For this review, take the finished solid that the model builds, in its own axes (mm). A direction names the side the tool comes from. Coordinates: 2 decimals unless noted, no trailing zeros. Write each loop counter-clockwise with the first axis right and the second up, starting at its lowest first coordinate (ties: lowest second). Pieces come first, ordered by that corner, then holes. Notation, with made-up numbers: (-36.5, 29.5) - (-28.5, 29.5) arc R19 ccw to (-28.5, 44.5) - close; hole circle Ø5 at (21, -39.75). An arc over 180 degrees is marked (long way). Use one line per item in the form item = value. Start each with the question number.
1) Tool access review of faces 1 (the flat face through (-1, -44, 8.875)), 2 (the flat face through (35, 35, 0)), 3 (the flat face through (-35, 35, 0)): name each direction out of +Z, -Z, +X, -X, +Y, -Y from which nothing blocks a thin tool from reaching the whole face with its end or side.
2) We need section B-B (y = -17.5). Give the boundary of the cut face in (x, z) (3 decimals).
3) We need section D-D (z = 22.5). Give the boundary of the cut face in (x, y) (3 decimals).
4) We need section A-A (x = 25). Give the boundary of the cut face in (y, z) (3 decimals).
5) We need section C-C (y = 17.5). Give the boundary of the cut face in (x, z) (3 decimals), plus the area to 4 significant figures.
6) For L1, parallel to X at y = 29, z = 0; L2, parallel to X at y = 17.5, z = 7.5 (3 decimals); L3, parallel to Y at x = -12, z = 0 (3 decimals), list the stretches that pass through material, from the lowest coordinate up. Write a range as from..to.
7) Mouldability with a two-part tool opening along X and no side actions: class faces 4 (the flat face through (50, -1, 0)), 5 (the cylindrical face through (-22.422, 28.406, -0.338)), 6 (the cylindrical face through (12.59, 80.78, 0.34)) as pulls with the +X half, pulls with the -X half, needs draft (parallel to the pull), parting line crosses it, or undercut.
8) Insertion check: P1, Ø6, axis at x = -25, y = 17.5, coming from the +Z side; P2, Ø1, axis at x = 10.5, z = 11, coming from the -Y side; P3, Ø4, axis at x = 21, z = -19, coming from the +Y side; P4, Ø9, axis at x = 14.5, y = -46.5, coming from the -Z side (3 decimals). Each pin has a flat end and moves straight along its axis. Give the tip position at first contact, or say it passes through.
```python
from build123d import *

# Parameters (mm, degrees)
SKETCH1_W               = 100
SKETCH1_H               = 70
BOSS_EXTRUDE1_DEPTH     = 25
CUT_EXTRUDE1_DEPTH      = 79.89866919
CUT_EXTRUDE1_DEPTH_BACK = 79.89866919
SKETCH2_R               = 4.875
CUT_EXTRUDE2_DEPTH      = 109.857705285
CUT_EXTRUDE2_DEPTH_BACK = 109.857705285
SKETCH3_R               = 4.875
SKETCH4_R               = 2.6
CUT_EXTRUDE4_DEPTH      = 20
SKETCH5_W               = 100
SKETCH5_H               = 17.75
BOSS_EXTRUDE2_DEPTH     = 20
FILLET1_R               = 2
SKETCH6_W               = 5
SKETCH6_H               = 50
BOSS_EXTRUDE3_DEPTH     = 50
CUT_EXTRUDE5_DEPTH      = 110.960291151
CUT_EXTRUDE5_DEPTH_BACK = 110.960291151
SKETCH7_R               = 2.65
FILLET2_R               = 5
FILLET3_R               = 2


with BuildPart() as part:
    # Sketch1 → Boss-Extrude1 (new, symmetric)
    with BuildSketch(Plane.XY):
        Rectangle(SKETCH1_W, SKETCH1_H)
    extrude(amount=BOSS_EXTRUDE1_DEPTH, both=True)

    # Sketch2 → Cut-Extrude1 (cut, two sides: drawn at the far end of the back side and taken through both)
    with BuildSketch(Plane.XY.offset(25).offset(-CUT_EXTRUDE1_DEPTH_BACK)):
        with Locations((25, 17.5)):
            Circle(SKETCH2_R)
        with Locations((-25, 17.5)):
            Circle(SKETCH2_R)
    extrude(amount=CUT_EXTRUDE1_DEPTH + CUT_EXTRUDE1_DEPTH_BACK, mode=Mode.SUBTRACT)

    # Sketch3 → Cut-Extrude2 (cut, two sides: drawn at the far end of the back side and taken through both)
    with BuildSketch(Plane.ZY.offset(50).offset(-CUT_EXTRUDE2_DEPTH_BACK)):
        with Locations((0, -17.5)):
            Circle(SKETCH3_R)
    extrude(amount=CUT_EXTRUDE2_DEPTH + CUT_EXTRUDE2_DEPTH_BACK, mode=Mode.SUBTRACT)

    # Sketch4 → Cut-Extrude4 (cut)
    with BuildSketch(Plane(origin=(0, 35, 0), x_dir=(1, 0, 0), z_dir=(0, 1, 0))):
        with Locations(Location((-25, 0, 0), (0, 0, 270))):
            Circle(SKETCH4_R)
        with Locations(Location((25, 0, 0), (0, 0, 270))):
            Circle(SKETCH4_R)
    extrude(amount=-CUT_EXTRUDE4_DEPTH, mode=Mode.SUBTRACT)

    # Sketch5 → Boss-Extrude2 (add)
    with BuildSketch(Plane.XZ.offset(35)):
        Rectangle(SKETCH5_W, SKETCH5_H)
    extrude(amount=BOSS_EXTRUDE2_DEPTH)

    # Fillet1
    fillet1_edges = [part.edges().sort_by_distance(p)[0] for p in [
        (0, -55, 8.875),
        (0, -55, -8.875),
    ]]
    fillet(fillet1_edges, radius=FILLET1_R)

    # Sketch6 → Boss-Extrude3 (add)
    with BuildSketch(Plane(origin=(0, 35, 0), x_dir=(1, 0, 0), z_dir=(0, 1, 0))):
        with Locations((-12.625, 0)):
            Rectangle(SKETCH6_W, SKETCH6_H)
        with Locations((12.625, 0)):
            Rectangle(SKETCH6_W, SKETCH6_H)
    extrude(amount=BOSS_EXTRUDE3_DEPTH)

    # Sketch7 → Cut-Extrude5 (cut, two sides: drawn at the far end of the back side and taken through both)
    with BuildSketch(Plane(origin=(15.125, 0, 0), x_dir=(0, 0, -1), z_dir=(1, 0, 0)).offset(-CUT_EXTRUDE5_DEPTH_BACK)):
        with Locations((0, 78.15)):
            Circle(SKETCH7_R)
    extrude(amount=CUT_EXTRUDE5_DEPTH + CUT_EXTRUDE5_DEPTH_BACK, mode=Mode.SUBTRACT)

    # Fillet2
    fillet2_edges = [part.edges().sort_by_distance(p)[0] for p in [
        (15.125, 35, 0),
        (10.125, 35, 0),
        (-15.125, 35, 0),
        (-10.125, 35, 0),
    ]]
    fillet(fillet2_edges, radius=FILLET2_R)

    # Fillet3
    fillet3_edges = [part.edges().sort_by_distance(p)[0] for p in [
        (15.125, 85, 0),
        (10.125, 85, 0),
        (-15.125, 85, 0),
        (-10.125, 85, 0),
    ]]
    fillet(fillet3_edges, radius=FILLET3_R)


solid = part.part
```
Determined:
q1.face_1 = +Z, +X, -X, -Y
q1.face_2 = +Z, -Z, +X, +Y
q1.face_3 = +Z, -Z, -X, +Y
q2.outline = (-50, -25) - (50, -25) - (50, -4.875) - (-50, -4.875) - close; (-50, 4.875) - (50, 4.875) - (50, 25) - (-50, 25) - close
q3.outline = (-50, -35) - (50, -35) - (50, 35) - (20.125, 35) arc R5 cw to (15.125, 40) - (15.125, 83) arc R2 ccw to (13.125, 85) - (12.125, 85) arc R2 ccw to (10.125, 83) - (10.125, 40) arc R5 cw to (5.125, 35) - (-5.125, 35) arc R5 cw to (-10.125, 40) - (-10.125, 83) arc R2 ccw to (-12.125, 85) - (-13.125, 85) arc R2 ccw to (-15.125, 83) - (-15.125, 40) arc R5 cw to (-20.125, 35) - (-50, 35) - close; hole circle Ø9.75 at (-25, 17.5); hole circle Ø9.75 at (25, 17.5)
q4.outline = (-55, -6.875) arc R2 ccw to (-53, -8.875) - (-35, -8.875) - (-35, -25) - (12.625, -25) - (12.625, 25) - (-35, 25) - (-35, 8.875) - (-53, 8.875) arc R2 ccw to (-55, 6.875) - close; (22.375, -25) - (35, -25) - (35, -2.6) - (22.375, -2.6) - close; (22.375, 2.6) - (35, 2.6) - (35, 25) - (22.375, 25) - close; hole circle Ø9.75 at (-17.5, 0)
q5.outline = (-50, -25) - (-29.875, -25) - (-29.875, 25) - (-50, 25) - close; (-20.125, -25) - (20.125, -25) - (20.125, 25) - (-20.125, 25) - close; (29.875, -25) - (50, -25) - (50, 25) - (29.875, 25) - close
q5.area = 4,025 mm²
q6.L1 = -50..-27.6, -22.4..22.4, 27.6..50
q6.L2 = -50..-29.875, -20.125..20.125, 29.875..50
q6.L3 = -55..-22.375, -12.625..75.5, 80.8..84.996
q7.face_4 = pulls with the +X half
q7.face_5 = undercut
q7.face_6 = needs draft
q8.P1 = through
q8.P2 = -35
q8.P3 = 35.13
q8.P4 = -8.875
